Design review of the part built by this model. Coordinates are the model's own, in mm. Round coordinates to 2 decimals unless told otherwise and drop trailing zeros. Order: outer loops, then holes, each group sorted by start corner. A loop starts at its lowest first (then second) coordinate and runs counter-clockwise, first axis right, second up. Notation, with made-up numbers: (49.5, 70.25) - (63.5, 70.25) arc R20 cw to (63.5, 81.25) - close; hole circle Ø4 at (89, 1.5). An arc over 180 degrees is marked (long way). Use CSV: the item, a comma, the result in double quotes.
from build123d import *

# Parameters (mm, degrees)
SCHIZZO1_R                   = 180.415
ESTRUSIONE_ESTRUSIONE1_DEPTH = 18
TAGLIO_ESTRUSIONE1_DEPTH     = 48
SCHIZZO1_18_R                = 7.5
TAGLIO_ESTRUSIONE2_DEPTH     = 80
TAGLIO_ESTRUSIONE3_DEPTH     = 135


with BuildPart() as part:
    # Schizzo1 → Estrusione-Estrusione1 (new body)
    with BuildSketch(Plane.XY):
        with Locations((-69.647392192, -18.728644796)):
            Circle(SCHIZZO1_R)
    extrude(amount=ESTRUSIONE_ESTRUSIONE1_DEPTH)

    # Schizzo1_17 → Taglio-Estrusione1 (cut)
    with BuildSketch(Plane.XY):
        with BuildLine():
            Line((44.382329363, 15.018559966), (26.382329363, 15.018559966))
            ThreePointArc((26.382329363, 15.018559966), (23.207329363, 18.193559966), (26.382329363, 21.368559966))
            Line((26.382329363, 21.368559966), (26.382329363, 26.668559966))
            ThreePointArc((26.382329363, 26.668559966), (23.207329363, 29.843559966), (26.382329363, 33.018559966))
            Line((26.382329363, 33.018559966), (44.382329363, 33.018559966))
            ThreePointArc((44.382329363, 33.018559966), (47.557329363, 29.843559966), (44.382329363, 26.668559966))
            Line((44.382329363, 26.668559966), (44.382329363, 21.368559966))
            ThreePointArc((44.382329363, 21.368559966), (47.557329363, 18.193559966), (44.382329363, 15.018559966))
        make_face()
    extrude(amount=TAGLIO_ESTRUSIONE1_DEPTH, mode=Mode.SUBTRACT)

    # Schizzo1_18 → Taglio-Estrusione2 (cut)
    with BuildSketch(Plane.XY):
        with Locations(Location((-220.074947502, 8.955026171, 0), (0, 0, 180))):
            Circle(SCHIZZO1_18_R)
    extrude(amount=TAGLIO_ESTRUSIONE2_DEPTH, mode=Mode.SUBTRACT)

    # Schizzo1_19 → Taglio-Estrusione3 (cut)
    with BuildSketch(Plane.XY):
        with BuildLine():
            Line((-66.997392192, -126.234256826), (-72.297392192, -126.234256826))
            ThreePointArc((-72.297392192, -126.234256826), (-75.472392192, -123.059256826), (-78.647392192, -126.234256826))
            Line((-78.647392192, -126.234256826), (-78.647392192, -137.234256826))
            Line((-78.647392192, -137.234256826), (-89.647392192, -137.234256826))
            ThreePointArc((-89.647392192, -137.234256826), (-92.822392192, -140.409256826), (-89.647392192, -143.584256826))
            Line((-89.647392192, -143.584256826), (-89.647392192, -148.884256826))
            ThreePointArc((-89.647392192, -148.884256826), (-92.822392192, -152.059256826), (-89.647392192, -155.234256826))
            Line((-89.647392192, -155.234256826), (-78.647392192, -155.234256826))
            Line((-78.647392192, -155.234256826), (-78.647392192, -166.234256826))
            ThreePointArc((-78.647392192, -166.234256826), (-75.472392192, -169.409256826), (-72.297392192, -166.234256826))
            Line((-72.297392192, -166.234256826), (-66.997392192, -166.234256826))
            ThreePointArc((-66.997392192, -166.234256826), (-63.822392192, -169.409256826), (-60.647392192, -166.234256826))
            Line((-60.647392192, -166.234256826), (-60.647392192, -155.234256826))
            Line((-60.647392192, -155.234256826), (-49.647392192, -155.234256826))
            ThreePointArc((-49.647392192, -155.234256826), (-46.472392192, -152.059256826), (-49.647392192, -148.884256826))
            Line((-49.647392192, -148.884256826), (-49.647392192, -143.584256826))
            ThreePointArc((-49.647392192, -143.584256826), (-46.472392192, -140.409256826), (-49.647392192, -137.234256826))
            Line((-49.647392192, -137.234256826), (-60.647392192, -137.234256826))
            Line((-60.647392192, -137.234256826), (-60.647392192, -126.234256826))
            ThreePointArc((-60.647392192, -126.234256826), (-63.822392192, -123.059256826), (-66.997392192, -126.234256826))
        make_face()
    extrude(amount=TAGLIO_ESTRUSIONE3_DEPTH, mode=Mode.SUBTRACT)


solid = part.part
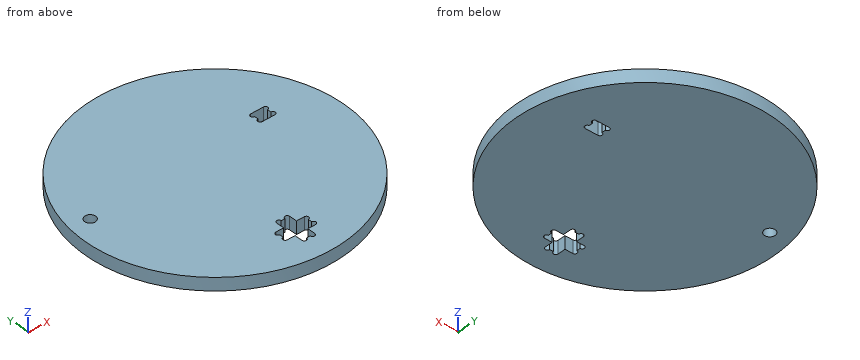
1) We need section A-A (z = 8.5). Give the number of separate pieces and of enclosed holes in the cut face, then the cut area to 3 significant figures.
Data:
separate pieces,"1"
enclosed holes,"3"
area,"100,000 mm2"
2) Insertion check: pin 1 Ø3 at (y, z) = (82.5, 5.5) entering from -X; pin 2 Ø3.5 at (x, z) = (-53, 7.5) entering from -Y; pin 3 Ø10 at (y, z) = (79, 10) entering from -X; pin 4 Ø6 at (x, y) = (-57.5, 105) entering from -Z. Each pin has a flat end and moves straight along its axis. Give the tip position at first contact, or say it passes through.
Data:
pin 1,"stops at x = -219.99"
pin 2,"stops at y = -198.53"
pin 3,"stops at x = -224.41"
pin 4,"stops at z = 0"
3) We need section C-C (x = -152). Give the boundary of the cut face in (y, z).
Data:
outline,"(-179.25, 0) - (141.79, 0) - (141.79, 18) - (-179.25, 18) - close"
4) To check wall thickness, follow L1, parallel to Y at x = 44.5, z = 13.25; L2, parallel to Y at x = -81.5, z = 4.75; L3, parallel to X at y = -159.5, z = 3. State the ranges of each line that lie inside material, in increasing order. Write a range as from..to.
Data:
L1,"y = -158.44..15.02, 21.37..26.67, 33.02..120.99"
L2,"y = -198.75..-155.23, -137.23..161.3"
L3,"x = -182.49..-78.65, -60.65..43.19"
5) We need section B-B (y = -99). Give the boundary of the cut face in (x, z).
Data:
outline,"(-231.22, 0) - (91.93, 0) - (91.93, 18) - (-231.22, 18) - close"
